Input: part model. Units: mm. Frame: model coordinates. A direction names the side the tool comes from. Give positions to 0.01 mm unless a question says otherwise; leave off trailing zeros. Loops run counter-clockwise (first coordinate to the right, second up) from the corner with the lowest first, then second, coordinate; pieces in that order, holes last. Notation, with made-up numbers: (82, 39.25) -> (123, 39.25) arc R14 ccw to (123, 53.25) -> close; hole circle Ø6 at (39.5, 85.5). An arc over 180 degrees is marked (long way). Answer in a Markdown table with one row per item. Add a question column.
Autodesk Inventor part; units mm, degrees
ref_plane "YZ Plane" through (0, 0, 0) normal (1, 0, 0) x (0, 1, 0)
ref_plane "XZ Plane" through (0, 0, 0) normal (0, 1, 0) x (-1, 0, 0)
ref_plane "XY Plane" through (0, 0, 0) normal (0, 0, 1) x (1, 0, 0)
sketch "Sketch1" plane through (0, 0, 0) normal (0, 1, 0) x (-1, 0, 0)
  line L0 (5.5, 7.5) -> (-5.5, 7.5)
  line L1 (-7.5, 5.5) -> (-7.5, -5.5)
  line L2 (-5.5, -7.5) -> (5.5, -7.5)
  line L3 (7.5, -5.5) -> (7.5, 5.5)
  line L4 (7.5, 7.5) -> (-7.5, -7.5) construction
  line L5 (-7.5, 7.5) -> (7.5, -7.5) construction
  arc A0 (7.5, 5.5) -> (5.5, 7.5) centre (5.5, 5.5) ccw
  arc A1 (-5.5, 7.5) -> (-7.5, 5.5) centre (-5.5, 5.5) ccw
  arc A2 (-7.5, -5.5) -> (-5.5, -7.5) centre (-5.5, -5.5) ccw
  arc A3 (5.5, -7.5) -> (7.5, -5.5) centre (5.5, -5.5) ccw
  line L6 (5.5, 4.5) -> (1, 4.5)
  line L7 (1, 4.5) -> (1, 1.5)
  line L8 (1, 1.5) -> (5.5, 1.5)
  line L9 (5.5, 1.5) -> (5.5, 4.5)
  line L10 (3.25, 0) -> (5.1677, 0)
  line L11 (0, 3.1331) -> (0, 1.6822) construction
  line L12 (5.5, -4.5) -> (1, -4.5)
  line L13 (1, -4.5) -> (1, -1.5)
  line L14 (1, -1.5) -> (5.5, -1.5)
  line L15 (5.5, -1.5) -> (5.5, -4.5)
  line L16 (-5.5, 4.5) -> (-1, 4.5)
  line L17 (-1, 4.5) -> (-1, 1.5)
  line L18 (-1, 1.5) -> (-5.5, 1.5)
  line L19 (-5.5, 1.5) -> (-5.5, 4.5)
  line L20 (-1, -4.5) -> (-1, -1.5)
  line L21 (-1, -1.5) -> (-5.5, -1.5)
  line L22 (-5.5, -1.5) -> (-5.5, -4.5)
  line L23 (-5.5, -4.5) -> (-1, -4.5)
  point P0 (0, 0)
  point P1 (5.5, -5.5)
  dimension "d0" = 2
  dimension "d1" = 11
  dimension "d2" = 11
  dimension "d5" = 3
  dimension "d6" = 4.5
  dimension "d7" = 2
  dimension "d8" = 3
extrude "Extrusion1" add sketch "Sketch1" along normal blind 3
properties part number "horn_base"
1) Pin query (flat end, axial travel): pin 1 (1 mm diameter, centred on x = -3, z = 0.5, fed in from -Y). Return the tip coordinate at first contact, or that it passes through.
2) Section C-C on x = -4.5. Output: boundary loops of the cut face in (y, z), and give its area (3 significant figures).
3) Reachability of faces 1 (the face through (0, 1, 7.5)), 2 (the face through (5.5, 1, -3)) from +Z, -Z, +X, -X, +Y, -Y: full face, straight path, thin tool, end or side. Return the list, or none.
4) Material intervals for line 1 along X through (y, z) = (1.8, -3); line 2 along Z through (x, y) = (4.5, 1.05); line 3 along X through (y, z) = (1.85, 6.75), sorted ascending.
5) Section D-D on z = 6.25. Output: boundary loops of the cut face in (x, y).
6) Section B-B on y = 0.4. Output: boundary loops of the cut face in (x, z), and give its area (3 significant figures).
7) Pull-direction query (Z, two-part tool) for faces 3 (the face through (-1, 1, -3)), 4 (the face through (0, 0, 0)), 5 (the face through (6.93, 1.48, 6.9)); classes: +Z half, -Z half, draft (parallel to the pull), parting line (faces both ways), or undercut.
8) Section A-A on z = -2. Output: boundary loops of the cut face in (x, y).
Working result:
| question | item | result |
|---|---|---|
| 1 | pin 1 | stops at y = 0 |
| 2 | outline | (0, -7.5) -> (3, -7.5) -> (3, -4.5) -> (0, -4.5) -> close; (0, -1.5) -> (3, -1.5) -> (3, 1.5) -> (0, 1.5) -> close; (0, 4.5) -> (3, 4.5) -> (3, 7.5) -> (0, 7.5) -> close |
| 2 | area | 27.0 mm2 |
| 3 | face 1 | +Z, +X, -X, +Y, -Y |
| 3 | face 2 | +Y, -Y |
| 4 | line 1 | x = -7.5 to -5.5, -1 to 1, 5.5 to 7.5 |
| 4 | line 2 | z = -7.5 to -4.5, -1.5 to 1.5, 4.5 to 7.5 |
| 4 | line 3 | x = -7.06 to 7.06 |
| 5 | outline | (-7.35, 0) -> (7.35, 0) -> (7.35, 3) -> (-7.35, 3) -> close |
| 6 | outline | (-7.5, -5.5) arc R2 ccw to (-5.5, -7.5) -> (5.5, -7.5) arc R2 ccw to (7.5, -5.5) -> (7.5, 5.5) arc R2 ccw to (5.5, 7.5) -> (-5.5, 7.5) arc R2 ccw to (-7.5, 5.5) -> close; hole (-5.5, -4.5) -> (-1, -4.5) -> (-1, -1.5) -> (-5.5, -1.5) -> close; hole (-5.5, 1.5) -> (-1, 1.5) -> (-1, 4.5) -> (-5.5, 4.5) -> close; hole (1, -4.5) -> (5.5, -4.5) -> (5.5, -1.5) -> (1, -1.5) -> close; hole (1, 1.5) -> (5.5, 1.5) -> (5.5, 4.5) -> (1, 4.5) -> close |
| 6 | area | 168 mm2 |
| 7 | face 3 | undercut |
| 7 | face 4 | draft |
| 7 | face 5 | +Z half |
| 8 | outline | (-7.5, 0) -> (-5.5, 0) -> (-5.5, 3) -> (-7.5, 3) -> close; (-1, 0) -> (1, 0) -> (1, 3) -> (-1, 3) -> close; (5.5, 0) -> (7.5, 0) -> (7.5, 3) -> (5.5, 3) -> close |
